Print and shaded views of the part. All mm, measured from the part's lowest x, y and z. A direction names the side the tool comes from. Round coordinates to 2 decimals unless told otherwise and drop trailing zeros. Loops run counter-clockwise (first coordinate to the right, second up) from the corner with the lowest first, then second, coordinate; pieces in that order, holes last. Notation, with made-up numbers: (-21.5, -1.75) - (32.5, -1.75) arc R14 cw to (32.5, 8.25) - close; hole circle Ø5 at (-18, 13). An arc over 180 degrees is marked (long way). Use one line per item in the form item = value.
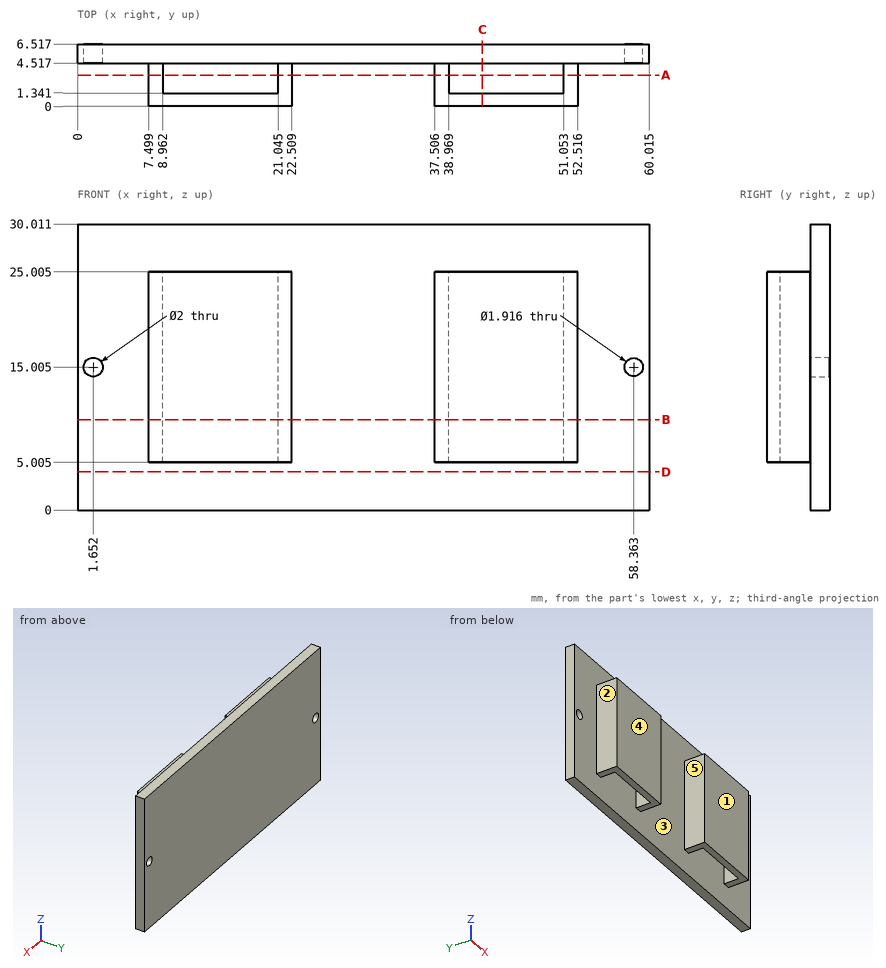
1. Cut at D-D, the plane z = 4. Give the cut face in (x, y) (1 decimal), plus the area to 3 significant figures.
Geometry check:
outline = (0, 4.5) - (60, 4.5) - (60, 6.5) - (0, 6.5) - close
area = 120 mm^2
2. Cut at C-C, the plane x = 42.5. Give the cut face in (y, z) (1 decimal).
Geometry check:
outline = (0, 5) - (1.3, 5) - (1.3, 25) - (0, 25) - close; (4.5, 0) - (6.5, 0) - (6.5, 30) - (4.5, 30) - close
3. Tool access for the marked faces 1 and 2: list every direction of +Z, -Z, +X, -X, +Y, -Y with a clear straight run to the whole face (end or side of a thin tool).
Geometry check:
face_1 = +Z, -Z, +X, -X, -Y
face_2 = +Z, -Z, -X, -Y
4. Cut at A-A, the plane y = 3.25. Give the cut face in (x, z) (1 decimal), plus the area to 3 significant figures.
Geometry check:
outline = (7.5, 5) - (9, 5) - (9, 25) - (7.5, 25) - close; (21, 5) - (22.5, 5) - (22.5, 25) - (21, 25) - close; (37.5, 5) - (39, 5) - (39, 25) - (37.5, 25) - close; (51.1, 5) - (52.5, 5) - (52.5, 25) - (51.1, 25) - close
area = 117 mm^2
5. Flat gauge pins, fed straight in: pin 1 (3.5 mm diameter, centred on x = 44.5, y = 2.5, fed in from +Z) (1 decimal); pin 2 (1 mm diameter, centred on x = 21.5, y = 3, fed in from -Z) (1 decimal); pin 3 (3.5 mm diameter, centred on y = 2, z = 15.5, fed in from -X); pin 4 (1.2 mm diameter, centred on x = 1.65, z = 15.01, fed in from -Y). Where does each tip first touch, or does it go through?
Geometry check:
pin_1 = 25
pin_2 = 5
pin_3 = 7.5
pin_4 = through
6. Pull direction Y, two halves, no side cores. Call the marked faces 3, 4 and 5: +Y half, -Y half, draft (parallel to the pull), parting line (faces both ways), or undercut.
Geometry check:
face_3 = undercut
face_4 = -Y half
face_5 = draft
7. Wall check: probe 1 along X at (y, z) = (2.5, 19.5) (1 decimal); probe 2 along Y at (x, z) = (40, 12); probe 3 along Y at (x, z) = (31.5, 3.5). Give the ranges that are in metal, low to high.
Geometry check:
probe_1 = 7.5 to 9, 21 to 22.5, 37.5 to 39, 51.1 to 52.5
probe_2 = 0 to 1.34, 4.52 to 6.52
probe_3 = 4.52 to 6.52
8. Cut at B-B, the plane z = 9.5. Give the cut face in (x, y) (1 decimal).
Geometry check:
outline = (0, 4.5) - (7.5, 4.5) - (7.5, 0) - (22.5, 0) - (22.5, 4.5) - (37.5, 4.5) - (37.5, 0) - (52.5, 0) - (52.5, 4.5) - (60, 4.5) - (60, 6.5) - (0, 6.5) - close; hole (9, 1.3) - (21, 1.3) - (21, 4.5) - (9, 4.5) - close; hole (39, 1.3) - (51.1, 1.3) - (51.1, 4.5) - (39, 4.5) - close
